Autodesk Inventor part; units mm, degrees
ref_plane "YZ Plane" through (0, 0, 0) normal (1, 0, 0) x (0, 1, 0)
ref_plane "XZ Plane" through (0, 0, 0) normal (0, 1, 0) x (-1, 0, 0)
ref_plane "XY Plane" through (0, 0, 0) normal (0, 0, 1) x (1, 0, 0)
sketch "スケッチ1" plane through (0, 0, 0) normal (0, 0, 1) x (1, 0, 0)
  line L0 (-16, -16) -> (16, -16)
  line L1 (16, -16) -> (16, 16)
  line L2 (16, 16) -> (-16, 16)
  line L3 (-16, 16) -> (-16, -16)
  line L4 (-16, -16) -> (16, 16) construction
  line L5 (16, -16) -> (-16, 16) construction
  line L6 (-14.4, 14.4) -> (14.4, 14.4)
  line L7 (14.4, 14.4) -> (14.4, -14.4)
  line L8 (14.4, -14.4) -> (-14.4, -14.4)
  line L9 (-14.4, -14.4) -> (-14.4, 14.4)
  point P0 (0, 0)
  dimension "d0" = 32
  dimension "d1" = 32
  dimension "d2" = 1.6
extrude "押し出し1" add sketch "スケッチ1" along normal blind 180
chamfer "面取り1" distance 32 angle 45 1 edges at (-16, 0, 0)
sketch "スケッチ2" plane through (16, -16, 180) normal (1, 0, 0) x (0, 0, -1)
  line L0 (0, 0) -> (0, 32)
  point P0 (180, 16)
  point P1 (131.5, 16)
  dimension "d8" = 131.5
hole "穴1" at (16, 0, 48.5) direction (-1, 0, 0) diameter 10.5 end through all
properties part number "PipeB"
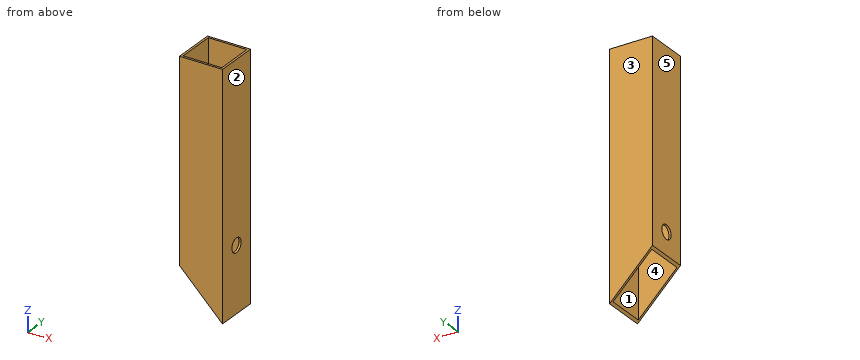
Check sheet for the modelled part. Datum: model origin and axes. Units: mm. Face numbers are marked on the shaded views. A direction names the side the tool comes from. Give positions to 0.01 mm unless a question says otherwise; leave off trailing zeros. Loops run counter-clockwise (first coordinate to the right, second up) from the corner with the lowest first, then second, coordinate; pieces in that order, holes last. Notation, with made-up numbers: M 83.25,-31.5 L 129.25,-31.5 A14 cw 129.25,-12.5 Z; hole C 46.5,-2 d2. An arc over 180 degrees is marked long. Answer as a JSON object with one key per item and string values. Group by question number.
Q1. Cross-section at A-A on y = 0. Record the cut outline in (x, z), then the cut area to 3 significant figures.
Q2. Access from +Z, -Z, +X, -X, +Y, -Y to the whole of each face (thin tool, end or side, straight path). Record for the marked faces 4 and 5.
Q3. Cross-section at B-B on x = -2. Record the cut outline in (y, z).
Q4. Cross-section at D-D on y = -7. Record the cut outline in (x, z).
Q5. Release check for a two-part mould opening along Y. For the marked faces 1, 2 and 3 record: released by +Y, released by -Y, zero draft, split by the parting line, or undercut.
Q6. Material ranges on line 1 along X through (y, z) = (-2, 140.5); line 2 along Y through (x, z) = (15, 48), recorded low to high. Write a range as [from, to].
Q7. Cross-section at C-C on z = 51. Record the cut outline in (x, y).
Q8. Go/stop test with a flat-tipped pin: P1, Ø2, axis at y = -1.5, z = 18, coming from the -X side. Record where the tip stops, or that it passes through.
Evaluation:
{
 "1": {"outline": "M -16,32 L -14.4,30.4 L -14.4,43.25 L -16,43.25 Z; M -16,53.75 L -14.4,53.75 L -14.4,180 L -16,180 Z; M 14.4,1.6 L 16,0 L 16,43.25 L 14.4,43.25 Z; M 14.4,53.75 L 16,53.75 L 16,180 L 14.4,180 Z", "area": "491 mm2"},
 "2": {"face 4": "+Z, -Z", "face 5": "+Z, -Z, -X, +Y, -Y"},
 "3": {"outline": "M -16,18 L -14.4,18 L -14.4,180 L -16,180 Z; M 14.4,18 L 16,18 L 16,180 L 14.4,180 Z"},
 "4": {"outline": "M -16,32 L -14.4,30.4 L -14.4,180 L -16,180 Z; M 14.4,1.6 L 16,0 L 16,180 L 14.4,180 Z"},
 "5": {"face 1": "undercut", "face 2": "zero draft", "face 3": "released by +Y"},
 "6": {"line 1": "x = [-16, -14.4], [14.4, 16]", "line 2": "y = [-16, -5.23], [5.23, 16]"},
 "7": {"outline": "M -16,-16 L 16,-16 L 16,-4.62 L 14.4,-4.62 L 14.4,-14.4 L -14.4,-14.4 L -14.4,-4.62 L -16,-4.62 Z; M -16,4.62 L -14.4,4.62 L -14.4,14.4 L 14.4,14.4 L 14.4,4.62 L 16,4.62 L 16,16 L -16,16 Z"},
 "8": {"P1": "stops at x = 14.4"}
}
